Part model, mm, in its own coordinate system. A direction names the side the tool comes from. Give positions to 0.01 mm unless a question says otherwise; leave off trailing zeros. Write each loop counter-clockwise with the first axis right and the second up, starting at its lowest first coordinate (ties: lowest second). Pieces come first, ordered by that corner, then holes.
```python
from build123d import *

# Parameters (mm, degrees)
SKETCH1_W                    = 90
SKETCH1_H                    = 100
BASE_FLANGE1_DEPTH           = 0.81
EDGE_FLANGE1_STRIP_W         = 4.7132
EDGE_FLANGE1_STRIP_H         = 0.81
EDGE_FLANGE1_STRIP_CUT_DEPTH = 90
EDGE_FLANGE1_DEPTH           = 90
EDGE_FLANGE2_DEPTH           = 48.4534
EDGE_FLANGE2_BEND_DEPTH      = 48.4534
EDGE_FLANGE3_DEPTH           = 99.2634
EDGE_FLANGE3_BEND_DEPTH      = 99.2634
CUT_EXTRUDE1_REACH           = 149.055


# Sheet-metal steps are written as plain solids
with BuildPart() as part:
    # Sketch1 → Base-Flange1 (new body)
    with BuildSketch(Plane(origin=(0, 0, 0), x_dir=(1, 0, 0), z_dir=(0, 1, 0))):
        with Locations((45, 50)):
            Rectangle(SKETCH1_W, SKETCH1_H)
    extrude(amount=-BASE_FLANGE1_DEPTH)

    # Edge-Flange1 strip (across the edge) → Edge-Flange1 strip cut (cut)
    with BuildSketch(Plane(origin=(90, 0, -100), x_dir=(0, 0, 1), z_dir=(-1, 0, 0))):
        with Locations((-1.62, -0.405)):
            Rectangle(EDGE_FLANGE1_STRIP_W, EDGE_FLANGE1_STRIP_H)
    extrude(amount=EDGE_FLANGE1_STRIP_CUT_DEPTH, mode=Mode.SUBTRACT)

    # Edge-Flange1 section (across the edge) → Edge-Flange1 (add)
    with BuildSketch(Plane(origin=(90, 0, -100), x_dir=(0, 0, 1), z_dir=(-1, 0, 0))):
        with BuildLine():
            Line((-0.81, 0.7366), (-0.81, 49.19))
            Line((-0.81, 49.19), (0, 49.19))
            Line((0, 49.19), (0, 0.7366))
            ThreePointArc((0, 0.7366), (0.215745145, 0.215745145), (0.7366, 0))
            Line((0.7366, 0), (0.7366, -0.81))
            ThreePointArc((0.7366, -0.81), (-0.357011348, -0.357011348), (-0.81, 0.7366))
        make_face()
    extrude(amount=EDGE_FLANGE1_DEPTH)

    # Edge-Flange2 section (across the edge) → Edge-Flange2 (add)
    with BuildSketch(Plane(origin=(-1.7366, 49.19, -100), x_dir=(1, 0, 0), z_dir=(0, -1, 0))):
        with BuildLine():
            Line((-0.81, 0.7366), (-0.81, 42.19))
            Line((-0.81, 42.19), (0, 42.19))
            Line((0, 42.19), (0, 0.7366))
            ThreePointArc((0, 0.7366), (0.215745145, 0.215745145), (0.7366, 0))
            Line((0.7366, 0), (1.7366, 0))
            Line((1.7366, 0), (1.7366, -0.81))
            Line((1.7366, -0.81), (0.7366, -0.81))
            ThreePointArc((0.7366, -0.81), (-0.357011348, -0.357011348), (-0.81, 0.7366))
        make_face()
    extrude(amount=EDGE_FLANGE2_DEPTH)

    # Edge-Flange2 section 2 (across the edge) → Edge-Flange2 bend (add)
    with BuildSketch(Plane(origin=(91.7366, 0.7366, -100), x_dir=(-1, 0, 0), z_dir=(0, 1, 0))):
        with BuildLine():
            Line((-0.81, 0.7366), (-0.81, 42.19))
            Line((-0.81, 42.19), (0, 42.19))
            Line((0, 42.19), (0, 0.7366))
            ThreePointArc((0, 0.7366), (0.215745145, 0.215745145), (0.7366, 0))
            Line((0.7366, 0), (1.7366, 0))
            Line((1.7366, 0), (1.7366, -0.81))
            Line((1.7366, -0.81), (0.7366, -0.81))
            ThreePointArc((0.7366, -0.81), (-0.357011348, -0.357011348), (-0.81, 0.7366))
        make_face()
    extrude(amount=EDGE_FLANGE2_BEND_DEPTH)

    # Edge-Flange3 section (across the edge) → Edge-Flange3 (add)
    with BuildSketch(Plane(origin=(-0.7366, 0, -99.2634), x_dir=(1, 0, 0), z_dir=(0, 0, 1))):
        with BuildLine():
            Line((-0.81, 0.7366), (-0.81, 49.19))
            Line((-0.81, 49.19), (0, 49.19))
            Line((0, 49.19), (0, 0.7366))
            ThreePointArc((0, 0.7366), (0.215745145, 0.215745145), (0.7366, 0))
            Line((0.7366, 0), (0.7366, -0.81))
            ThreePointArc((0.7366, -0.81), (-0.357011348, -0.357011348), (-0.81, 0.7366))
        make_face()
    extrude(amount=EDGE_FLANGE3_DEPTH)

    # Edge-Flange3 section 2 (across the edge) → Edge-Flange3 bend (add)
    with BuildSketch(Plane(origin=(90.7366, 0, 0), x_dir=(-1, 0, 0), z_dir=(0, 0, -1))):
        with BuildLine():
            Line((-0.81, 0.7366), (-0.81, 49.19))
            Line((-0.81, 49.19), (0, 49.19))
            Line((0, 49.19), (0, 0.7366))
            ThreePointArc((0, 0.7366), (0.215745145, 0.215745145), (0.7366, 0))
            Line((0.7366, 0), (0.7366, -0.81))
            ThreePointArc((0.7366, -0.81), (-0.357011348, -0.357011348), (-0.81, 0.7366))
        make_face()
    extrude(amount=EDGE_FLANGE3_BEND_DEPTH)

    # Cut-Extrude1: up to this face of the body (flat: up to its plane)
    cut_extrude1_end = Plane(part.part.faces().sort_by_distance((92.5466, 24.9633, -78.5367))[0])
    # Sketch23 → Cut-Extrude1 (cut, up to the picked face)
    with BuildSketch(Plane.ZY.offset(2.5466), mode=Mode.PRIVATE) as cut_extrude1_sk1:
        Polygon((-99.2634, 49.19), (-57.81, 0.7366), (0, 0.7366), (0, 49.19), align=None)
    cut_extrude1_tool1 = split(extrude(cut_extrude1_sk1.sketch, amount=-CUT_EXTRUDE1_REACH, mode=Mode.PRIVATE), bisect_by=cut_extrude1_end, keep=Keep.BOTH, mode=Mode.PRIVATE)
    add(cut_extrude1_tool1.solids().sort_by(Axis((-2.5466, 27.094531, -40.180017), (1, 0, 0)))[0], mode=Mode.SUBTRACT)


solid = part.part
```
1) Saw through at B-B, the plane x = 42.5. Write the cut outline in (y, z), then the cut area to 3 significant figures.
Answers follow:
outline: (-0.81, -99.26) arc R1.55 ccw to (0.74, -100.81) - (49.19, -100.81) - (49.19, -100) - (0.74, -100) arc R0.74 cw to (0, -99.26) - (0, 0) - (-0.81, 0) - close
area: 121 mm2
2) Wall check: L1, parallel to X at y = 18, z = -79; L2, parallel to Y at x = 47.5, z = -12; L3, parallel to Z at x = 62.5, y = 17. Give the ranges that are in metal, low to high.
Answers follow:
L1: x = -2.55 to -1.74, -1.55 to -0.74, 90.74 to 91.55, 91.74 to 92.55
L2: y = -0.81 to 0
L3: z = -100.81 to -100
3) Saw through at A-A, the plane y = 40.5. Write the cut outline in (x, z).
Answers follow:
outline: (-2.55, -99.26) arc R1.55 ccw to (-1, -100.81) - (91, -100.81) arc R1.55 ccw to (92.55, -99.26) - (92.55, -91.83) - (91.74, -91.83) - (91.74, -99.26) arc R0.74 cw to (91, -100) - (-1, -100) arc R0.74 cw to (-1.74, -99.26) - (-1.74, -91.83) - (-2.55, -91.83) - close; (-1.55, -99.26) - (-0.74, -99.26) - (-0.74, -91.83) - (-1.55, -91.83) - close; (90.74, -99.26) - (91.55, -99.26) - (91.55, -91.83) - (90.74, -91.83) - close
4) Pin check, flat tips, straight feed: pin 1 Ø0.8 at (y, z) = (0, -100.5) entering from -X; pin 2 Ø1.5 at (x, y) = (46, 21) entering from +Z; pin 3 Ø0.8 at (y, z) = (0, -100) entering from +X. Stop position of each tip, or through.
Answers follow:
pin 1: stops at x = 0
pin 2: stops at z = -100
pin 3: stops at x = 90
5) Saw through at C-C, the plane z = -60. Write the cut outline in (x, y).
Answers follow:
outline: (-2.55, 0.74) - (-1.74, 0.74) - (-1.74, 3.3) - (-2.55, 3.3) - close; (-1.55, 0.74) arc R1.55 ccw to (0, -0.81) - (90, -0.81) arc R1.55 ccw to (91.55, 0.74) - (91.55, 3.3) - (90.74, 3.3) - (90.74, 0.74) arc R0.74 cw to (90, 0) - (0, 0) arc R0.74 cw to (-0.74, 0.74) - (-0.74, 3.3) - (-1.55, 3.3) - close; (91.74, 0.74) - (92.55, 0.74) - (92.55, 3.3) - (91.74, 3.3) - close
6) Saw through at D-D, the plane z = -33. Write the cut outline in (x, y).
Answers follow:
outline: (-1.55, 0.74) arc R1.55 ccw to (0, -0.81) - (90, -0.81) arc R1.55 ccw to (91.55, 0.74) - (90.74, 0.74) arc R0.74 cw to (90, 0) - (0, 0) arc R0.74 cw to (-0.74, 0.74) - close
7) Two-plate mould, pull along X, no slides. Class faces 4 (the face through (-1.737, 15, -87)), 5 (the face through (-2.547, 15, -88)), 6 (the face through (91.136, 25.302, -78.827)): +X half, -X half, draft (parallel to the pull), parting line (faces both ways), or undercut.
Answers follow:
face 4: undercut
face 5: -X half
face 6: draft
8) 3-axis set-ups, long thin cutter, end or side, ignore diameter. For faces 1 (the face through (-0.737, 15, -88)), 2 (the face through (-2.147, 25.302, -78.827)), 3 (the face through (91.547, 14, -87)): which of +Z, -Z, +X, -X, +Y, -Y reach the whole face in a straight line?
Answers follow:
face 1: +Z, +Y
face 2: +Z, +X, -X, +Y
face 3: +Z, +Y, -Y
